Autodesk Inventor part; units mm, degrees
ref_plane "YZ Plane" through (0, 0, 0) normal (1, 0, 0) x (0, 1, 0)
ref_plane "XZ Plane" through (0, 0, 0) normal (0, 1, 0) x (-1, 0, 0)
ref_plane "XY Plane" through (0, 0, 0) normal (0, 0, 1) x (1, 0, 0)
sketch "Boceto1" plane through (0, 0, 0) normal (0, 1, 0) x (-1, 0, 0)
  line L0 (-53, -53) -> (53, -53)
  line L1 (53, -53) -> (53, 53)
  line L2 (53, 53) -> (-53, 53)
  line L3 (-53, 53) -> (-53, -53)
  line L4 (-53, -53) -> (53, 53) construction
  line L5 (53, -53) -> (-53, 53) construction
  point P0 (0, 0)
  dimension "d0" = 106
  dimension "d1" = 106
extrude "Extrusión1" add sketch "Boceto1" along normal blind 185
shell "Vaciado1" thickness 1.5 removed faces 2 at (17.6667, 0, -17.6667) at (17.6667, 185, -17.6667)
split "Dividir1" plane through (0, 0, 0) removes the side toward (1, 0, 0)
sketch "Boceto2" plane through (-51.5, 0, -51.5) normal (1, 0, 0) x (0, 0, -1)
  line L0 (-71.9943, 102) -> (-31.0057, 102)
  line L1 (-31.0057, 102) -> (-31.0057, 73)
  line L2 (-31.0057, 102) -> (-2.0057, 102) construction
  line L3 (-31.0057, 73) -> (-71.9943, 73)
  line L4 (-71.9943, 73) -> (-71.9943, 102)
  line L5 (-31.0057, 102) -> (-32.0057, 102)
  line L6 (-32.0057, 102) -> (-71.0057, 102)
  line L7 (-71.0057, 102) -> (-71.0057, 73)
  line L8 (-71.0057, 73) -> (-32.0057, 73)
  line L9 (-32.0057, 73) -> (-32.0057, 102)
  point P0 (-51.5, 0)
  dimension "d5" = 29
  dimension "d6" = 90
  dimension "d8" = 1
  dimension "d9" = 39
  dimension "d10" = 29
extrude "Extrusión2" cut sketch "Boceto2" against normal blind 10 contours L0 L9 L3 L7
properties part number "Caja"
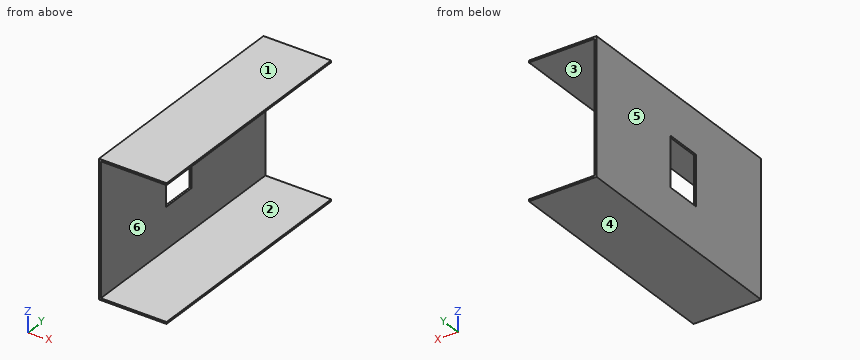
For this review, take the finished solid that the model builds, in its own axes (mm). Face numbers are marked on the shaded views. A direction names the side the tool comes from. Coordinates: 2 decimals unless noted, no trailing zeros. Loops run counter-clockwise (first coordinate to the right, second up) from the corner with the lowest first, then second, coordinate; pieces in that order, holes last. Notation, with made-up numbers: (-0.75, 48) -> (47.25, 48) arc R9 ccw to (47.25, 53) -> close; hole circle Ø1 at (6, 11.5). An arc over 180 degrees is marked (long way). Write each question's results on one line, items separated by ' | '.
Q1. Add section A-A, the plane z = -4.5. State the section outline as (x, y) points.
Taken from the geometry:
outline: (-53, 0) -> (-51.5, 0) -> (-51.5, 73) -> (-53, 73) -> close; (-53, 102) -> (-51.5, 102) -> (-51.5, 185) -> (-53, 185) -> close
Q2. Add section D-D, the plane z = -42. State the section outline as (x, y) points.
Taken from the geometry:
outline: (-53, 0) -> (-51.5, 0) -> (-51.5, 185) -> (-53, 185) -> close
Q3. Add section B-B, the plane y = 98. State the section outline as (x, z) points.
Taken from the geometry:
outline: (-53, -53) -> (0, -53) -> (0, -51.5) -> (-51.5, -51.5) -> (-51.5, -19.49) -> (-53, -19.49) -> close; (-53, 19.51) -> (-51.5, 19.51) -> (-51.5, 51.5) -> (0, 51.5) -> (0, 53) -> (-53, 53) -> close
Q4. Mouldability with a two-part tool opening along Z and no side actions: class the marked faces 3, 4, 5 and 6 as +Z half, -Z half, draft (parallel to the pull), parting line (faces both ways), or undercut.
Taken from the geometry:
face 3: undercut | face 4: -Z half | face 5: draft | face 6: undercut
Q5. To check wall thickness, follow line 1 along Z through (x, y) = (-9.5, 56); line 2 along X through (y, z) = (124, 15). State the ranges of each line that lie inside material, in increasing order. Write a range as [from, to].
Taken from the geometry:
line 1: [-53, -51.5], [51.5, 53] | line 2: [-53, -51.5]
Q6. Machinability: for the marked faces 1 and 2, which of the approach directions +Z, -Z, +X, -X, +Y, -Y give a long, thin tool a straight path to every point of the face, cutting with its end or side? Answer none if there is none.
Taken from the geometry:
face 1: +Z, +X, -X, +Y, -Y | face 2: +X, +Y, -Y
Q7. Add section C-C, the plane x = -6. State the section outline as (y, z) points.
Taken from the geometry:
outline: (0, -53) -> (185, -53) -> (185, -51.5) -> (0, -51.5) -> close; (0, 51.5) -> (185, 51.5) -> (185, 53) -> (0, 53) -> close
Q8. For pin 1 Ø10 at (y, z) = (98, -14.5) entering from -X; pin 2 Ø3 at (y, z) = (76, -2) entering from +X, all flat-tipped, find the tip position at first contact; note any pin that passes through.
Taken from the geometry:
pin 1: x = -53 | pin 2: through
